The listing builds one solid part. Answer for the finished solid, in the listing's coordinates (mm). Coordinates: 2 decimals unless noted, no trailing zeros. Order: outer loops, then holes, each group sorted by start corner. A loop starts at its lowest first (then second) coordinate and runs counter-clockwise, first axis right, second up. Notation, with made-up numbers: (6, 63.25) -> (49, 63.25) arc R10 ccw to (49, 82.25) -> close; hole circle Ø9 at (-6, 17). An arc over 180 degrees is marked (long way). Put each result on its own line as item: value. Start each with the question number.
```python
from build123d import *

# Parameters (mm, degrees)
F0_W     = 50
F0_H     = 50
F0_W_2   = 46
F0_H_2   = 46
F1_DEPTH = 1200
F3_DEPTH = 50
F4_DEPTH = 50


with BuildPart() as f1:
    # F0 (on Front) → F1 (new body)
    with BuildSketch(Plane.XZ):
        with Locations((25, 25)):
            Rectangle(F0_W, F0_H)
        with Locations((25, 25)):
            Rectangle(F0_W_2, F0_H_2, mode=Mode.SUBTRACT)
    extrude(amount=F1_DEPTH)

    # F2 (on face) → F3 (cut)
    with BuildSketch(Plane.XY.offset(50)):
        Polygon((50, 0), (0, 0), (0, -50), align=None)
    extrude(amount=-F3_DEPTH, mode=Mode.SUBTRACT)

    # F2 (on face) → F4 (cut)
    with BuildSketch(Plane.XY.offset(50)):
        Polygon((50, 0), (0, 0), (0, -50), align=None)
        Polygon((0, -1150), (0, -1200), (50, -1200), align=None)
    extrude(amount=-F4_DEPTH, mode=Mode.SUBTRACT)


solid = f1.part
```
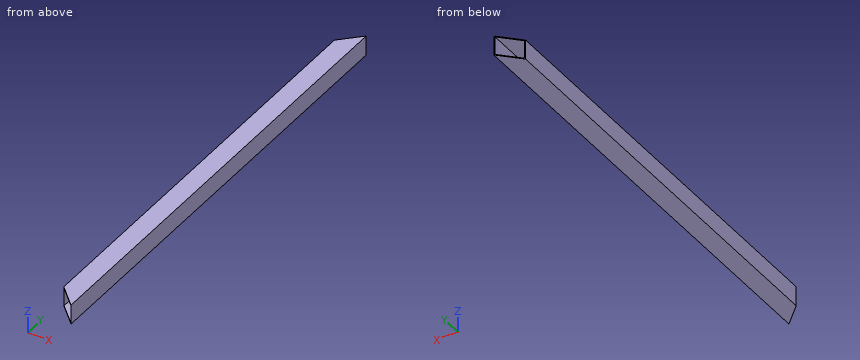
(1) The part is cut by section C-C on y = -701. Determine the outline of the cut face in (x, z), plus the area to 3 significant figures.
(2) Find the intervals of material crossed by L1, parallel to X at y = -996, z = 7, in increasing order.
(3) The part is cut by section A-A on x = 19. Determine the outline of the cut face in (y, z), plus the area to 3 significant figures.
(4) The part is cut by section B-B on z = 17.5. Determine the outline of the cut face in (x, y), plus the area to 3 significant figures.
Worked out:
1. outline: (0, 0) -> (50, 0) -> (50, 50) -> (0, 50) -> close; hole (2, 2) -> (48, 2) -> (48, 48) -> (2, 48) -> close
1. area: 384 mm2
2. L1: 0 to 2, 48 to 50
3. outline: (-1169, 0) -> (-31, 0) -> (-31, 2) -> (-1169, 2) -> close; (-1169, 48) -> (-31, 48) -> (-31, 50) -> (-1169, 50) -> close
3. area: 4,550 mm2
4. outline: (0, -1150) -> (2, -1152) -> (2, -48) -> (0, -50) -> close; (48, -1198) -> (50, -1200) -> (50, 0) -> (48, -2) -> close
4. area: 4,600 mm2
